```python
from build123d import *

# Parameters (mm, degrees)
BOSS_EXTRUDE1_DEPTH = 5
CAVITY1_START       = -38.899371069
CAVITY1_OUTLINE_W   = 5
CAVITY1_OUTLINE_H   = 5
CAVITY1_DEPTH       = 6.666666666


# Read off the part's stored shape, not the designer's step: Cavity1
with BuildPart() as part:
    # Sketch1 → Boss-Extrude1 (new body)
    with BuildSketch(Plane.XY):
        Polygon((3.333333333, -50), (10, -50), (10, 50), (-10, 50), (-10, -50), (-3.333333333, -50), (-3.333333333, -45), (3.333333333, -45), align=None)
    extrude(amount=BOSS_EXTRUDE1_DEPTH)

    # Cavity1 outline → Cavity1 (cut)
    with BuildSketch(Plane(origin=(0, 0, 0), x_dir=(1, 0, 0), z_dir=(0, 1, 0)).offset(CAVITY1_START)):
        with Locations((0, -2.5)):
            Rectangle(CAVITY1_OUTLINE_W, CAVITY1_OUTLINE_H)
    extrude(amount=CAVITY1_DEPTH, mode=Mode.SUBTRACT)


solid = part.part
```
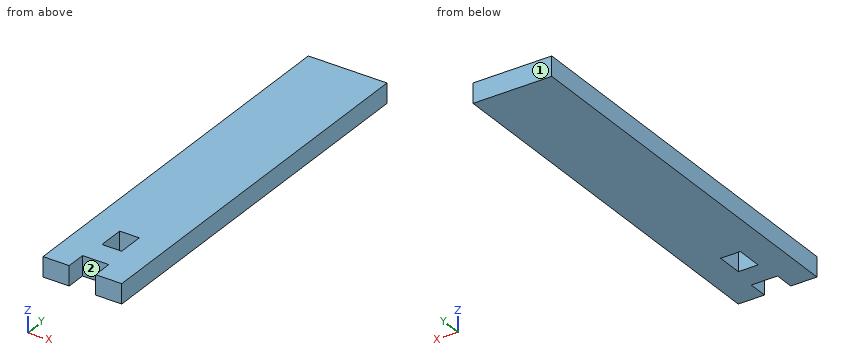
The model under review builds one solid part; all positions refer to its coordinate system, in mm. Face numbers are marked on the shaded views. A direction names the side the tool comes from. Give positions to 0.01 mm unless a question says otherwise; leave off trailing zeros. Loops run counter-clockwise (first coordinate to the right, second up) from the corner with the lowest first, then second, coordinate; pieces in that order, holes last. Notation, with made-up numbers: (8, 13.25) - (15, 13.25) arc R19 ccw to (15, 44.25) - close; hole circle Ø10 at (89.25, -20). An arc over 180 degrees is marked (long way). Answer as a JSON object with one key per item and string values.
Q1. To check wall thickness, follow line 1 along Y through (x, z) = (0.25, 1.95); line 2 along X through (y, z) = (-37.5, 1.6); line 3 along Y through (x, z) = (-2.75, 0.2). State the ranges of each line that lie inside material, in increasing order.
Worked out:
{"line 1": "y = -45 to -38.9, -32.23 to 50", "line 2": "x = -10 to -2.5, 2.5 to 10", "line 3": "y = -45 to 50"}
Q2. For the marked faces 1 and 2, list the 3-axis set-ups (+Z, -Z, +X, -X, +Y, -Y) from which the entire face can be reached by the end or side of a thin tool; tool diameter is ignored.
Worked out:
{"face 1": "+Z, -Z, +X, -X, +Y", "face 2": "+Z, -Z, -Y"}
Q3. Add section A-A on y = -38. State the section outline as (x, z) points.
Worked out:
{"outline": "(-10, 0) - (-2.5, 0) - (-2.5, 5) - (-10, 5) - close; (2.5, 0) - (10, 0) - (10, 5) - (2.5, 5) - close"}
Q4. Add section B-B on z = 4.15. State the section outline as (x, y) points, plus the area to 3 significant figures.
Worked out:
{"outline": "(-10, -50) - (-3.33, -50) - (-3.33, -45) - (3.33, -45) - (3.33, -50) - (10, -50) - (10, 50) - (-10, 50) - close; hole (-2.5, -38.9) - (2.5, -38.9) - (2.5, -32.23) - (-2.5, -32.23) - close", "area": "1,930 mm^2"}
